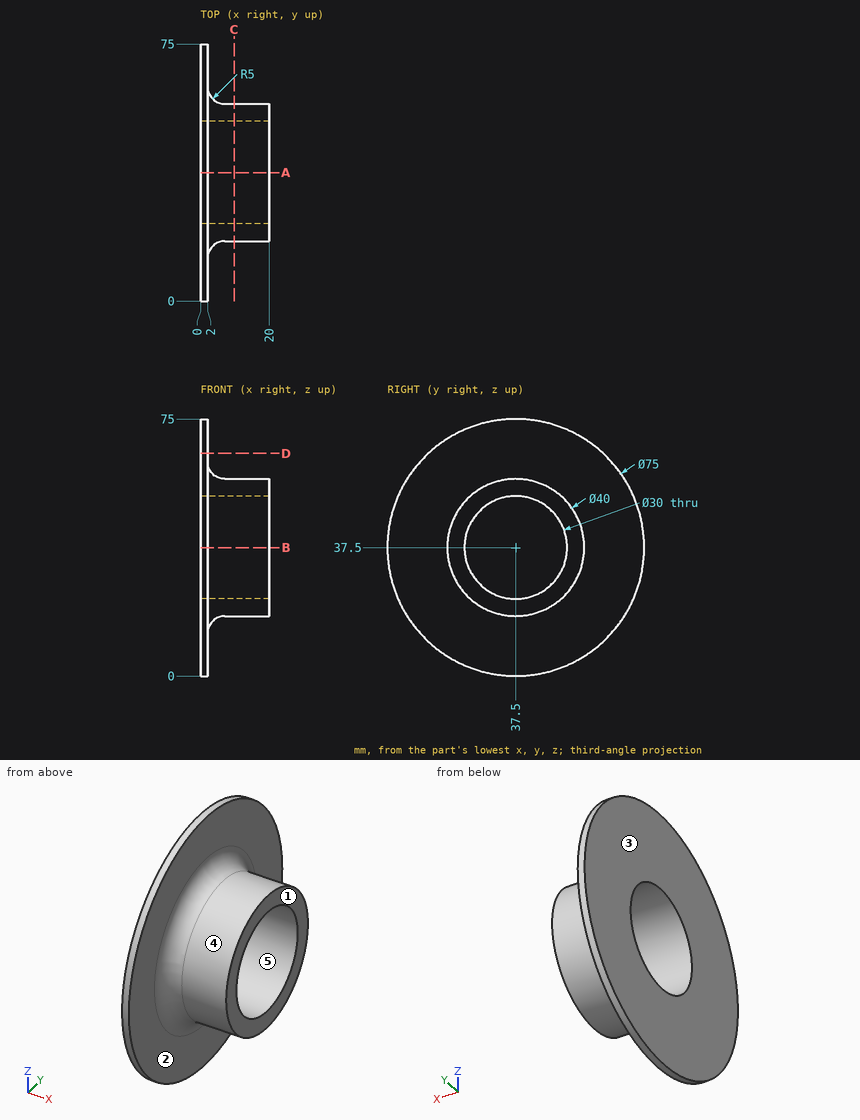
Drawing for the job (mm, zero at the part's lowest x, y, z). A direction names the side the tool comes from. Round coordinates to 2 decimals unless told otherwise and drop trailing zeros. Write each loop counter-clockwise with the first axis right and the second up, starting at its lowest first coordinate (ties: lowest second). Pieces come first, ordered by that corner, then holes. Notation, with made-up numbers: M 50,-4.75 L 104,-4.75 A14 ccw 104,0.25 Z; hole C 80.25,75.5 d10. An arc over 180 degrees is marked long. Answer as a JSON object with one key per item and string values. Group by question number.
(1) Cut at A-A (y = 37.5). Give the cut face in (x, z).
(2) Cut at D-D (z = 65). Give the cut face in (x, y).
(3) Cut at C-C (x = 9.75). Give the cut face in (y, z), and give its area (3 significant figures).
(4) Mould opens along Z. For the marked faces 3, 4 and 5 say: pulls with the +Z half, pulls with the -Z half, needs draft (parallel to the pull), parting line crosses it, or undercut.
(5) Which spindle directions (+Z, -Z, +X, -X, +Y, -Y) get a long thin tool onto all of the face, cutting with end or side? Do the marked faces 1 and 2. Say none if no direction does.
(6) Drill centre lines: L1, parallel to Z at x = 11.25, y = 37.5; L2, parallel to X at y = 72.5, z = 41; L3, parallel to Z at x = 18.25, y = 41. Where is each one in solid material? Low to high.
(7) Flat gauge pins, fed straight in: pin 1 (1.5 mm diameter, centred on y = 24.5, z = 56.5, fed in from -X); pin 2 (1 mm diameter, centred on x = 3.5, z = 54, fed in from +Y); pin 3 (1 mm diameter, centred on x = 16.5, y = 45.5, fed in from -Z); pin 4 (10 mm diameter, centred on x = 12, y = 17, fed in from -Z). Where does each tip first touch, or does it go through?
Responses:
{
 "1": {"outline": "M 0,0 L 2,0 L 2,12.5 A5 cw 7,17.5 L 20,17.5 L 20,22.5 L 0,22.5 Z; M 0,52.5 L 20,52.5 L 20,57.5 L 7,57.5 A5 cw 2,62.5 L 2,75 L 0,75 Z"},
 "2": {"outline": "M 0,12 L 2,12 L 2,63 L 0,63 Z"},
 "3": {"outline": "C 37.5,37.5 d40; hole C 37.5,37.5 d30", "area": "550 mm2"},
 "4": {"face 3": "needs draft", "face 4": "parting line crosses it", "face 5": "undercut"},
 "5": {"face 1": "+Z, -Z, +X, +Y, -Y", "face 2": "+X"},
 "6": {"L1": "z = 17.5 to 22.5, 52.5 to 57.5", "L2": "x = 0 to 2", "L3": "z = 17.81 to 22.91, 52.09 to 57.19"},
 "7": {"pin 1": "stops at x = 0", "pin 2": "stops at y = 52.2", "pin 3": "stops at z = 18.96", "pin 4": "stops at z = 24.86"}
}
